from build123d import *

# Parameters (mm, degrees)
SKETCH1_R           = 27
SKETCH1_R_2         = 2.8
BOSS_EXTRUDE2_DEPTH = 4
SKETCH2_R           = 27
SKETCH2_R_2         = 2.8
SKETCH2_R_3         = 1.5
BOSS_EXTRUDE3_DEPTH = 5
SKETCH3_R           = 3
BOSS_EXTRUDE4_DEPTH = 25
SKETCH4_R           = 12.2
SKETCH4_R_2         = 7.64
BOSS_EXTRUDE5_DEPTH = 3


with BuildPart() as part:
    # Sketch1 → Boss-Extrude2 (new body)
    with BuildSketch(Plane(origin=(0, 0, 0), x_dir=(0, 0, -1), z_dir=(1, 0, 0))):
        Circle(SKETCH1_R)
        Circle(SKETCH1_R_2, mode=Mode.SUBTRACT)
    extrude(amount=BOSS_EXTRUDE2_DEPTH)

    # Sketch2 → Boss-Extrude3 (add)
    with BuildSketch(Plane(origin=(4, 0, 0), x_dir=(0, 0, -1), z_dir=(1, 0, 0))):
        Circle(SKETCH2_R)
        Circle(SKETCH2_R_2, mode=Mode.SUBTRACT)
        Circle(SKETCH2_R_2)
        Circle(SKETCH2_R_3, mode=Mode.SUBTRACT)
    extrude(amount=BOSS_EXTRUDE3_DEPTH)

    # Sketch3 → Boss-Extrude4 (add)
    with BuildSketch(Plane(origin=(9, 0, 0), x_dir=(0, 0, -1), z_dir=(1, 0, 0))):
        with Locations((0, 20)):
            Circle(SKETCH3_R)
        with Locations((17.320508076, -10)):
            Circle(SKETCH3_R)
        with Locations((-17.320508076, -10)):
            Circle(SKETCH3_R)
    extrude(amount=BOSS_EXTRUDE4_DEPTH)

    # Sketch4 → Boss-Extrude5 (add)
    with BuildSketch(Plane(origin=(9, 0, 0), x_dir=(0, 0, -1), z_dir=(1, 0, 0))):
        Circle(SKETCH4_R)
        Circle(SKETCH4_R_2, mode=Mode.SUBTRACT)
    extrude(amount=BOSS_EXTRUDE5_DEPTH)


solid = part.part
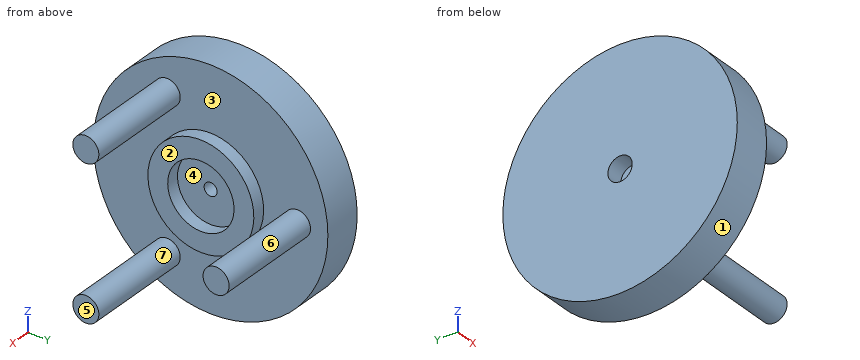
CAD build for the part. Positions are in the model's coordinates, mm. Face numbers are marked on the shaded views. A direction names the side the tool comes from. Coordinates: 2 decimals unless noted, no trailing zeros. Order: outer loops, then holes, each group sorted by start corner. A loop starts at its lowest first (then second) coordinate and runs counter-clockwise, first axis right, second up.
Item 1: Band-saw the part on B-B on z = 0. List the corners of the cut face in (x, y), plus the area to 3 significant figures.
Check sheet entries:
outline: (0, -27) - (9, -27) - (9, -12.2) - (12, -12.2) - (12, -7.64) - (9, -7.64) - (9, -1.5) - (4, -1.5) - (4, -2.8) - (0, -2.8) - close; (0, 2.8) - (4, 2.8) - (4, 1.5) - (9, 1.5) - (9, 7.64) - (12, 7.64) - (12, 12.2) - (9, 12.2) - (9, 17) - (34, 17) - (34, 23) - (9, 23) - (9, 27) - (0, 27) - close
area: 626 mm2
Item 2: Two-plate mould, pull along Z, no slides. Class the marked faces 4, 5, 6 and 7: +Z half, -Z half, draft (parallel to the pull), parting line (faces both ways), or undercut.
Check sheet entries:
face 4: undercut
face 5: draft
face 6: parting line
face 7: undercut
Item 3: Band-saw the part on D-D on y = 20. List the corners of the cut face in (x, z).
Check sheet entries:
outline: (0, -18.14) - (9, -18.14) - (9, -3) - (34, -3) - (34, 3) - (9, 3) - (9, 18.14) - (0, 18.14) - close
Item 4: 3-axis set-ups, long thin cutter, end or side, ignore diameter. For the marked faces 1, 2 and 3: which of +Z, -Z, +X, -X, +Y, -Y reach the whole face in a straight line?
Check sheet entries:
face 1: +X, -X
face 2: +X, -Y
face 3: +X
Item 5: Drill centre lines: L1, parallel to Y at x = 11.35, z = 0; L2, parallel to Y at x = 7.9, z = 0; L3, parallel to Y at x = 1, z = 0. Where is each one in solid material? Low to high.
Check sheet entries:
L1: y = -12.2 to -7.64, 7.64 to 12.2, 17 to 23
L2: y = -27 to -1.5, 1.5 to 27
L3: y = -27 to -2.8, 2.8 to 27
Item 6: Pin check, flat tips, straight feed: pin 1 Ø17.5 at (y, z) = (0, 0) entering from -X; pin 2 Ø17 at (y, z) = (2.5, 0) entering from +X; pin 3 Ø5 at (x, y) = (23, -6.5) entering from -Z; pin 4 Ø1 at (x, z) = (28.5, -21) entering from -Y. Stop position of each tip, or through.
Check sheet entries:
pin 1: stops at x = 0
pin 2: stops at x = 12
pin 3: stops at z = -20.15
pin 4: passes through
Item 7: Band-saw the part on A-A on y = 0. List the corners of the cut face in (x, z).
Check sheet entries:
outline: (0, -27) - (9, -27) - (9, -12.2) - (12, -12.2) - (12, -7.64) - (9, -7.64) - (9, -1.5) - (4, -1.5) - (4, -2.8) - (0, -2.8) - close; (0, 2.8) - (4, 2.8) - (4, 1.5) - (9, 1.5) - (9, 7.64) - (12, 7.64) - (12, 12.2) - (9, 12.2) - (9, 27) - (0, 27) - close
Item 8: Band-saw the part on C-C on x = 15. List the corners of the cut face in (y, z), plus the area to 3 significant figures.
Check sheet entries:
outline: circle Ø6 at (-10, -17.32); circle Ø6 at (-10, 17.32); circle Ø6 at (20, 0)
area: 84.8 mm2
